Could you check a few things on this drawing? It's one solid part, dimensions in mm from its lowest x, y, z. Give positions to 0.01 mm unless a question says otherwise; leave off trailing zeros. Order: outer loops, then holes, each group sorted by start corner. A loop starts at its lowest first (then second) coordinate and runs counter-clockwise, first axis right, second up. Notation, with made-up numbers: (69.5, 62) - (128.5, 62) arc R30 ccw to (128.5, 93) - close; hole circle Ø3 at (9.25, -2). An arc over 180 degrees is marked (long way). One line per question, with ' | ' between items. Start each with the question number.
1. Imagine slicing it at C-C (x = 34.5). Please give me the cut outline in (y, z).
2. If we mould it in two halves opening along X, with no side actions, what happens to the marked faces 1, 2 and 3? For each: released by +X, released by -X, zero draft, split by the parting line, or undercut.
3. Imagine slicing it at A-A (y = 20.5). Please give me the cut outline in (x, z) (1 decimal), and give its area (3 significant figures).
4. For P1, Ø1.1, axis at x = 44, y = 7.5, coming from the +Z side; P2, Ø2, axis at y = 20.5, z = 10.5, coming from the +X side; P3, Ø3.5, axis at x = 36, y = 12.5, coming from the +Z side; P4, Ø12, axis at x = 12, y = 3, coming from the -Z side, each with a flat end and sliding along its axis, tell me the tip position at first contact or that it passes through.
5. I need wall thicknesses on probe 1 along Z at (x, y) = (39.5, 11); probe 2 along X at (y, z) = (19.75, 17) (1 decimal); probe 3 along X at (y, z) = (1, 15) (1 decimal). Which ranges of each line are inside material? Lowest first, please. Write a range as from..to.
6. Imagine slicing it at D-D (z = 21). Please give me the cut outline in (x, y).
7. Imagine slicing it at B-B (z = 4.5). Please give me the cut outline in (x, y) (1 decimal).
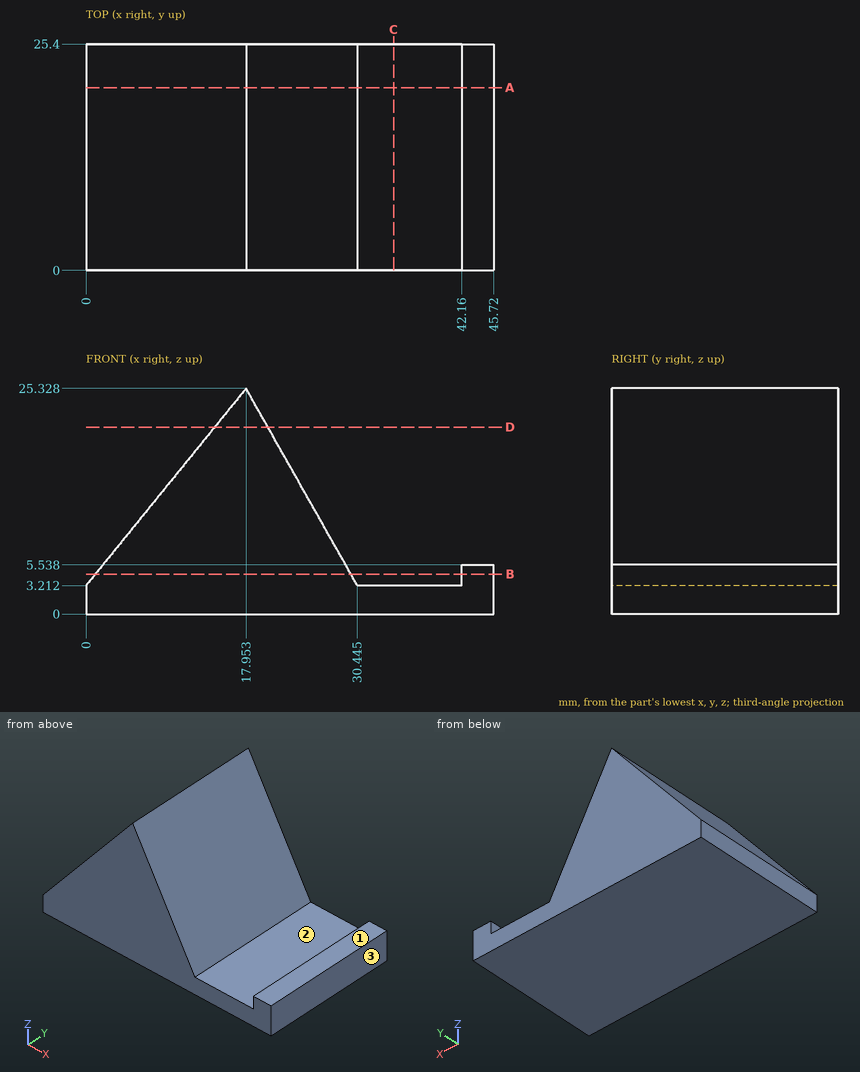
Results found:
1) outline: (0, 0) - (25.4, 0) - (25.4, 3.21) - (0, 3.21) - close
2) face 1: zero draft | face 2: undercut | face 3: released by +X
3) outline: (0, 0) - (45.7, 0) - (45.7, 5.5) - (42.2, 5.5) - (42.2, 3.2) - (30.4, 3.2) - (18, 25.3) - (0, 3.2) - close | area: 492 mm2
4) P1: stops at z = 5.54 | P2: stops at x = 26.89 | P3: stops at z = 3.21 | P4: stops at z = 0
5) probe 1: z = 0..3.21 | probe 2: x = 11.2..22.7 | probe 3: x = 9.6..23.8
6) outline: (14.44, 0) - (20.4, 0) - (20.4, 25.4) - (14.44, 25.4) - close
7) outline: (1, 0) - (29.7, 0) - (29.7, 25.4) - (1, 25.4) - close; (42.2, 0) - (45.7, 0) - (45.7, 25.4) - (42.2, 25.4) - close
